from build123d import *

# Parameters (mm, degrees)
SKETCH1_R           = 49.276
BOSS_EXTRUDE1_DEPTH = 12.7
SKETCH1_10_R        = 28.952599956
CUT_EXTRUDE2_DEPTH  = 13.7
SKETCH2_R           = 12.7
CUT_EXTRUDE3_DEPTH  = 13.7
CUT_EXTRUDE4_DEPTH  = 6.35
CIRPATTERN1_COUNT   = 4


with BuildPart() as part:
    # Sketch1 → Boss-Extrude1 (new body)
    with BuildSketch(Plane(origin=(0, 0, 0), x_dir=(1, 0, 0), z_dir=(0, 1, 0))):
        Circle(SKETCH1_R)
    extrude(amount=BOSS_EXTRUDE1_DEPTH)

    # Sketch1<10> → Cut-Extrude2 (cut, through all)
    with BuildSketch(Plane(origin=(0, 0, 0), x_dir=(1, 0, 0), z_dir=(0, 1, 0))):
        Circle(SKETCH1_10_R)
    extrude(amount=CUT_EXTRUDE2_DEPTH, mode=Mode.SUBTRACT)

    # Sketch2 → Cut-Extrude3 (cut, through all)
    with BuildSketch(Plane(origin=(0, 12.7, 0), x_dir=(1, 0, 0), z_dir=(0, 1, 0))):
        with Locations((49.276, 0)):
            Circle(SKETCH2_R)
    extrude(amount=-CUT_EXTRUDE3_DEPTH, mode=Mode.SUBTRACT)

    # Sketch3 → Cut-Extrude4 (cut)
    with BuildSketch(Plane(origin=(0, 12.7, 0), x_dir=(1, 0, 0), z_dir=(0, 1, 0))):
        with BuildLine():
            ThreePointArc((-33.582072771, 36.060623461), (-34.84339375, 34.84339375), (-36.060623461, 33.582072771))
            Line((-36.060623461, 33.582072771), (-21.674311893, 19.195761203))
            ThreePointArc((-21.674311893, 19.195761203), (-20.472579762, 20.472579762), (-19.195761203, 21.674311893))
            Line((-19.195761203, 21.674311893), (-33.582072771, 36.060623461))
        make_face()
        with BuildLine():
            ThreePointArc((-19.195761203, 21.674311893), (-20.472579762, 20.472579762), (-21.674311893, 19.195761203))
            Line((-21.674311893, 19.195761203), (-19.199787587, 16.721236897))
            Line((-19.199787587, 16.721236897), (-16.721236897, 19.199787587))
            Line((-16.721236897, 19.199787587), (-19.195761203, 21.674311893))
        make_face()
        with BuildLine():
            Line((-19.199787587, 16.721236897), (-21.674311893, 19.195761203))
            ThreePointArc((-21.674311893, 19.195761203), (-10.264632547, -27.071947896), (28.952599956, 0))
            ThreePointArc((28.952599956, 0), (11.884566657, 26.400949218), (-19.195761203, 21.674311893))
            Line((-19.195761203, 21.674311893), (-16.721236897, 19.199787587))
            Line((-16.721236897, 19.199787587), (-19.199787587, 16.721236897))
        make_face()
        with BuildLine():
            Line((-34.897275286, 37.375825976), (-37.375825976, 34.897275286))
            Line((-37.375825976, 34.897275286), (-36.060623461, 33.582072771))
            ThreePointArc((-36.060623461, 33.582072771), (-34.84339375, 34.84339375), (-33.582072771, 36.060623461))
            Line((-33.582072771, 36.060623461), (-34.897275286, 37.375825976))
        make_face()
    cut_extrude4 = extrude(amount=-CUT_EXTRUDE4_DEPTH, mode=Mode.SUBTRACT)

    # CirPattern1: Cut-Extrude4 ×4 about axis
    cirpattern1_axis = Axis((0, 0, 0), (0, 1, 0))
    for i in range(1, CIRPATTERN1_COUNT):
        add(cut_extrude4.rotate(cirpattern1_axis, i * 360 / CIRPATTERN1_COUNT), mode=Mode.SUBTRACT)


solid = part.part
Source: CAD feature listing. Evaluate the final solid. Frame: model axes, mm. A direction names the side the tool comes from. Give positions to 0.01 mm unless a question says otherwise; leave off trailing zeros. Write each loop counter-clockwise with the first axis right and the second up, starting at its lowest first coordinate (ties: lowest second). Pieces come first, ordered by that corner, then holes. Notation, with made-up numbers: M 19,-22.75 L 77,-22.75 A18 cw 77,-4.75 Z; hole C 2.25,39.5 d6. An arc over 180 degrees is marked long. Answer as a JSON object with one key per item and string values.
Q1. Ray query, line 1 along X through (y, z) = (5.5, 0); line 2 along Z through (x, y) = (0, 8.5); line 3 along Z through (x, y) = (-30.5, 11.25). Return the intervals inside material, ascending.
Geometry check:
{"line 1": "x = -49.28 to -28.95, 28.95 to 36.58", "line 2": "z = -49.28 to -28.95, 28.95 to 49.28", "line 3": "z = -38.7 to -32.98, -28.02 to 28.02, 32.98 to 38.7"}
Q2. Cut plane D-D, the plane y = 3.25. Return the cut outline in (x, z).
Geometry check:
{"outline": "M 47.64,-12.59 A12.7 cw 47.64,12.59 A49.28 ccw long Z; hole C 0,0 d57.91"}
Q3. Contact query for flat-ended pins moving along their axis: P1, Ø5, axis at x = -33, y = 9.5, coming from the -Z side; P2, Ø1, axis at y = 10.5, z = -14.5, coming from the -X side; P3, Ø1.5, axis at x = 26, y = 6.5, coming from the +Z side (3 decimals). Output: stop coordinate, or through.
Geometry check:
{"P1": "stops at z = -38.7", "P2": "stops at x = -47.25", "P3": "stops at z = 42.315"}
Q4. Mould query, pull axis Z, two halves, no side actions, for faces 1 (the face through (36.58, 6.44, -0.26)), 2 (the face through (28.77, 9.57, -26.29)), 3 (the face through (34, 12.7, 0)), 4 (the face through (-49.236, 6.261, -1.988)). Classes: +Z half, -Z half, draft (parallel to the pull), parting line (faces both ways), or undercut.
Geometry check:
{"face 1": "undercut", "face 2": "undercut", "face 3": "draft", "face 4": "parting line"}
Q5. Access query for faces 5 (the face through (28, 6.35, 27)), 6 (the face through (0, 12.7, 35)). Directions: +Z, -Z, +X, -X, +Y, -Y. A direction counts if a zero-diameter tool reaches every point of the face in a straight line with its end or side. Return the directions, or none.
Geometry check:
{"face 5": "+Y", "face 6": "+Z, -Z, +X, -X, +Y"}
Q6. Cut plane C-C, the plane x = 0. Return the cut outline in (y, z).
Geometry check:
{"outline": "M 0,-49.28 L 12.7,-49.28 L 12.7,-28.95 L 0,-28.95 Z; M 0,28.95 L 12.7,28.95 L 12.7,49.28 L 0,49.28 Z"}
Q7. Cut plane A-A, the plane z = 0. Return the cut outline in (x, y), then the cut area to 3 significant figures.
Geometry check:
{"outline": "M -49.28,0 L -28.95,0 L -28.95,12.7 L -49.28,12.7 Z; M 28.95,0 L 36.58,0 L 36.58,12.7 L 28.95,12.7 Z", "area": "355 mm^2"}
Q8. Cut plane B-B, the plane y = 8.5. Return the cut outline in (x, z), then the cut area to 3 significant figures.
Geometry check:
{"outline": "M -36.06,-33.58 L -21.67,-19.2 A28.95 cw -21.67,19.2 L -36.06,33.58 A49.28 ccw Z; M -33.58,-36.06 A49.28 ccw 33.58,-36.06 L 19.2,-21.67 A28.95 cw -19.2,-21.67 Z; M -33.58,36.06 L -19.2,21.67 A28.95 cw 19.2,21.67 L 33.58,36.06 A49.28 ccw Z; M 21.67,-19.2 L 36.06,-33.58 A49.28 ccw 47.64,-12.59 A12.7 cw 47.64,12.59 A49.28 ccw 36.06,33.58 L 21.67,19.2 A28.95 cw Z", "area": "4,470 mm^2"}
